Autodesk Inventor part; units mm, degrees
ref_plane "YZ Plane" through (0, 0, 0) normal (1, 0, 0) x (0, 1, 0)
ref_plane "XZ Plane" through (0, 0, 0) normal (0, 1, 0) x (-1, 0, 0)
ref_plane "XY Plane" through (0, 0, 0) normal (0, 0, 1) x (1, 0, 0)
sketch "スケッチ1" plane through (0, 0, 0) normal (0, 0, 1) x (1, 0, 0)
  circle A0 centre (0, 0) radius 3
  dimension "d20" = 6
extrude "押し出し1" add sketch "スケッチ1" along normal blind 3
sketch "スケッチ2" plane through (0, 0, 3) normal (0, 0, 1) x (1, 0, 0)
  circle A0 centre (0, 0) radius 2.25
  dimension "d3" = 4.5
extrude "押し出し2" add sketch "スケッチ2" along normal blind 4
sketch "スケッチ5" plane through (0, 0, 7) normal (0, 0, 1) x (1, 0, 0)
  point P0 (0, 0)
  point P1 (0, 0)
hole "穴2" at (0, 0, 7) direction (0, 0, -1) diameter 2.5 end through all
properties part number "RD009"
The listing builds one solid part. Answer for the finished solid, in the listing's coordinates (mm). Round coordinates to 2 decimals unless told otherwise and drop trailing zeros. Loops run counter-clockwise (first coordinate to the right, second up) from the corner with the lowest first, then second, coordinate; pieces in that order, holes last. Notation, with made-up numbers: (-7, 30) - (41, 30) arc R22 cw to (41, 64) - close; hole circle Ø5 at (52, 85). An arc over 180 degrees is marked (long way). Return JSON: item names as keys, results as strings. Group by question number.
1. Each of these flat-tipped pins is pushed along its axis until it touches: P1, Ø2, axis at x = 0, y = 0, coming from the -Z side; P2, Ø1.5, axis at y = 1, z = 5, coming from the +X side; P3, Ø2, axis at x = 1.5, z = 1, coming from the +Y side; P4, Ø1.5, axis at x = 1, z = 1, coming from the -Y side. Where does it stop, or does it pass through?
2. The part is cut by section A-A on y = 0. Determine the outline of the cut face in (x, z).
3. The part is cut by section C-C on z = 3.25. Determine the outline of the cut face in (x, y).
4. The part is cut by section D-D on y = -2. Determine the outline of the cut face in (x, z), then the cut area to 3 significant figures.
5. The mould has two halves that part along X. Classify faces 1 (the cylindrical face through (1.22, 0.27, 3.45)), 2 (the cylindrical face through (-0.29, -2.23, 4.97)), 3 (the flat face through (1, -1, 0)): pulls with the +X half, pulls with the -X half, needs draft (parallel to the pull), parting line crosses it, or undercut.
6. Consider probe 1 along Y at (x, z) = (0, 2.25); probe 2 along Y at (x, z) = (0, 4.5); probe 3 along Z at (x, y) = (-2.35, 1.3). Determine where each line is inside the solid, lowest interval first.
Resolved:
{
 "1": {"P1": "passes through", "P2": "stops at x = 2.24", "P3": "stops at y = 2.96", "P4": "stops at y = -2.99"},
 "2": {"outline": "(-3, 0) - (-1.25, 0) - (-1.25, 7) - (-2.25, 7) - (-2.25, 3) - (-3, 3) - close; (1.25, 0) - (3, 0) - (3, 3) - (2.25, 3) - (2.25, 7) - (1.25, 7) - close"},
 "3": {"outline": "circle Ø4.5 at (0, 0); hole circle Ø2.5 at (0, 0)"},
 "4": {"outline": "(-2.24, 0) - (2.24, 0) - (2.24, 3) - (1.03, 3) - (1.03, 7) - (-1.03, 7) - (-1.03, 3) - (-2.24, 3) - close", "area": "21.7 mm²"},
 "5": {"face 1": "undercut", "face 2": "parting line crosses it", "face 3": "needs draft"},
 "6": {"probe 1": "y = -3 to -1.25, 1.25 to 3", "probe 2": "y = -2.25 to -1.25, 1.25 to 2.25", "probe 3": "z = 0 to 3"}
}
